Input: part model. Units: mm. Frame: model coordinates. Face numbers are marked on the shaded views. Give positions to 0.01 mm unless a question says otherwise; leave off trailing zeros. Loops run counter-clockwise (first coordinate to the right, second up) from the corner with the lowest first, then second, coordinate; pieces in that order, holes last.
from build123d import *

# Parameters (mm, degrees)
SKETCH032_R     = 12.4
PAD022_DEPTH    = 10
SKETCH033_R     = 11.4
POCKET009_DEPTH = 9
SKETCH034_R     = 8.4
POCKET010_DEPTH = 5


with BuildPart() as part:
    # Sketch032 → Pad022 (new body)
    with BuildSketch(Plane.XY):
        with Locations((0, 18)):
            Circle(SKETCH032_R)
    extrude(amount=PAD022_DEPTH)

    # Sketch033 (on Face2 of Pad022) → Pocket009 (cut)
    with BuildSketch(Plane(origin=(0, 0, 0), x_dir=(1, 0, 0), z_dir=(0, 0, -1))):
        with Locations((0, -18)):
            Circle(SKETCH033_R)
    extrude(amount=-POCKET009_DEPTH, mode=Mode.SUBTRACT)

    # Sketch034 (on Face5 of Pocket009) → Pocket010 (cut)
    with BuildSketch(Plane(origin=(0, 0, 9), x_dir=(1, 0, 0), z_dir=(0, 0, -1))):
        with Locations((0, -18)):
            Circle(SKETCH034_R)
    extrude(amount=-POCKET010_DEPTH, mode=Mode.SUBTRACT)


with BuildPart() as part_1:
    # Body039 placement: moved
    add(part.part.moved(Location((0, 0, 11))))


solid = part_1.part
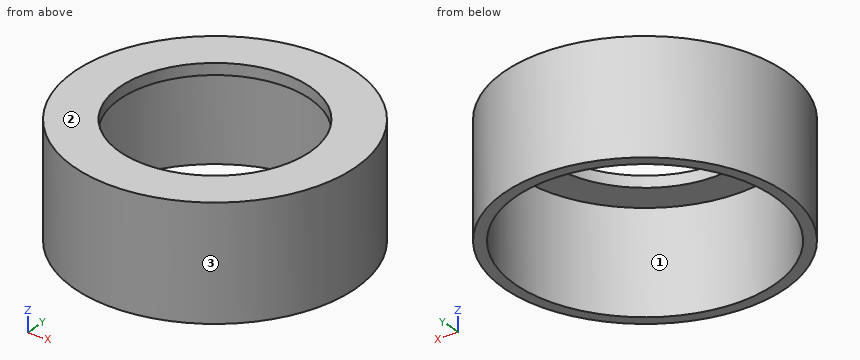
(1) Cut plane C-C (z = 14.5). Return the cut outline in (x, y).
Values follow:
outline: circle Ø24.8 at (0, 18); hole circle Ø22.8 at (0, 18)
(2) Ray query, probe 1 along Y at (x, z) = (0, 20.75); probe 2 along Y at (x, z) = (0, 14.75); probe 3 along Z at (x, y) = (-2, 7.75). Return the intervals inside material, ascending.
Values follow:
probe 1: y = 5.6 to 9.6, 26.4 to 30.4
probe 2: y = 5.6 to 6.6, 29.4 to 30.4
probe 3: z = 20 to 21
(3) Cut plane B-B (x = 0). Return the cut outline in (y, z), and give its area (3 significant figures).
Values follow:
outline: (5.6, 11) - (6.6, 11) - (6.6, 20) - (9.6, 20) - (9.6, 21) - (5.6, 21) - close; (26.4, 20) - (29.4, 20) - (29.4, 11) - (30.4, 11) - (30.4, 21) - (26.4, 21) - close
area: 26.0 mm2
(4) Mould query, pull axis Y, two halves, no side actions, for the marked faces 1, 2 and 3. Classes: +Y half, -Y half, draft (parallel to the pull), parting line (faces both ways), or undercut.
Values follow:
face 1: undercut
face 2: draft
face 3: parting line
(5) Cut plane A-A (y = 18). Return the cut outline in (x, z), and give its area (3 significant figures).
Values follow:
outline: (-12.4, 11) - (-11.4, 11) - (-11.4, 20) - (-8.4, 20) - (-8.4, 21) - (-12.4, 21) - close; (8.4, 20) - (11.4, 20) - (11.4, 11) - (12.4, 11) - (12.4, 21) - (8.4, 21) - close
area: 26.0 mm2
(6) Pin query (flat end, axial travel): pin 1 Ø10 at (x, y) = (0, 18) entering from +Z; pin 2 Ø6 at (y, z) = (22, 14) entering from +X; pin 3 Ø1.5 at (x, z) = (0.5, 13) entering from -Y; pin 4 Ø1 at (x, z) = (6.5, 18.5) entering from +Y. Return the tip coordinate at first contact, or that it passes through.
Values follow:
pin 1: passes through
pin 2: stops at x = 12.36
pin 3: stops at y = 5.6
pin 4: stops at y = 28.85
(7) Cut plane D-D (y = 7.75). Return the cut outline in (x, z).
Values follow:
outline: (-6.98, 11) - (-4.99, 11) - (-4.99, 20) - (4.99, 20) - (4.99, 11) - (6.98, 11) - (6.98, 21) - (-6.98, 21) - close
